Work out the finished part from the listing and answer in its coordinate system (mm). Face numbers are marked on the shaded views. A direction names the side the tool comes from. Coordinates: 2 decimals unless noted, no trailing zeros. Order: outer loops, then holes, each group sorted by start corner. A loop starts at its lowest first (then second) coordinate and runs counter-clockwise, first axis right, second up. Notation, with made-up numbers: (-20.5, 10) - (6.5, 10) arc R6 ccw to (6.5, 14) - close; hole circle Ø5 at (59.5, -39.5). An arc over 180 degrees is marked (long way). Answer as a JSON object with one key per item and string values. Group by question number.
1) A tool of negligible diameter and unlimited length cuts with its end or side. For the marked faces 1 and 2, from which of +Z, -Z, +X, -X, +Y, -Y can it reach the whole face along a straight path? Write none if from no direction.
2) Section B-B (y = -17) is taken. Give the vertices of the cut face in (x, z) (3 decimals), plus the area to 3 significant figures.
3) Each of these flat-tipped pins is pushed along its axis until it touches: P1, Ø6, axis at x = 3.5, y = -8.5, coming from the -Z side; P2, Ø5, axis at x = -1.5, y = -12, coming from the -Z side (3 decimals); P3, Ø6, axis at y = -9.5, z = 0, coming from the +X side (3 decimals). Where does it stop, or does it pass through?
4) Section A-A (z = 0) is taken. Give the vertices of the cut face in (x, y) (3 decimals), plus the area to 3 significant figures.
5) Find the intervals of material crossed by line 1 along Y through (x, z) = (4.25, 2.5) (3 decimals); line 2 along X through (y, z) = (-22.5, 5.5); line 3 along Z through (x, y) = (0.25, -6), in increasing order.
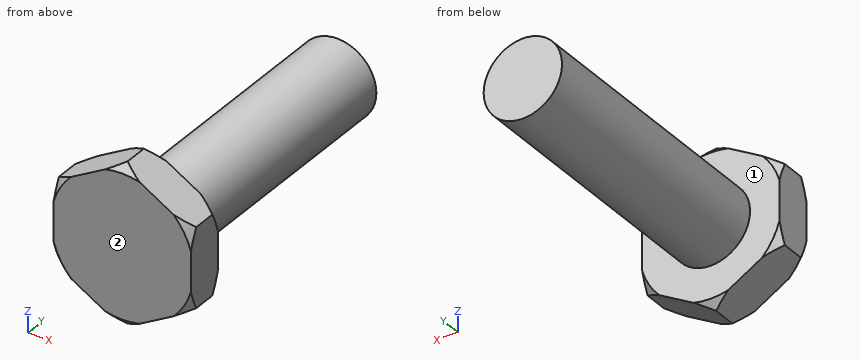
from build123d import *

# Parameters (mm, degrees)
F0_R     = 3.175
F1_DEPTH = 22.225
F2_R     = 3.175
F3_DEPTH = 3.175


with BuildPart() as f1:
    # F0 (on Front) → F1 (new body)
    with BuildSketch(Plane.XZ):
        Circle(F0_R)
    extrude(amount=F1_DEPTH)

    # F2 (on face) → F3 (join)
    with BuildSketch(Plane.XZ.offset(22.225)):
        Polygon((5.5626, 3.2115686074), (0, 6.4231372148), (-5.5626, 3.2115686074), (-5.5626, -3.2115686074), (0, -6.4231372148), (5.5626, -3.2115686074), align=None)
        Circle(F2_R, mode=Mode.SUBTRACT)
        Circle(F2_R)
    extrude(amount=F3_DEPTH)

    # F4 (on Right) → F5 (revolve, cut)
    with BuildSketch(Plane.YZ):
        Polygon((-24.765, 6.4231372148), (-25.4, 6.4231372148), (-25.4, 5.7881372148), align=None)
        Polygon((-22.225, 5.7881372148), (-22.225, 6.4231372148), (-22.86, 6.4231372148), align=None)
    revolve(axis=Axis((0, 0, 0), (0, 1, 0)), mode=Mode.SUBTRACT)


solid = f1.part
Report:
{
 "1": {"face 1": "+Y", "face 2": "+Z, -Z, +X, -X, -Y"},
 "2": {"outline": "circle Ø6.35 at (0, 0)", "area": "31.7 mm²"},
 "3": {"P1": "stops at z = -3.14", "P2": "stops at z = -3.175", "P3": "stops at x = 3.175"},
 "4": {"outline": "(-5.563, -25.4) - (5.563, -25.4) - (5.563, -22.225) - (3.175, -22.225) - (3.175, 0) - (-3.175, 0) - (-3.175, -22.225) - (-5.563, -22.225) - close", "area": "176 mm²"},
 "5": {"line 1": "y = -25.4 to -22.225", "line 2": "x = -1.6 to 1.6", "line 3": "z = -3.17 to 3.17"}
}
